Verification items for the finished model (mm, model axes). A direction names the side the tool comes from. Round coordinates to 2 decimals unless told otherwise and drop trailing zeros. Write each loop counter-clockwise with the first axis right and the second up, starting at its lowest first coordinate (ties: lowest second). Pieces come first, ordered by that corner, then holes. Notation, with made-up numbers: M 10,-11 L 56,-11 A20 ccw 56,24 Z; hole C -26,-35.75 d5. An arc over 180 degrees is marked long. Use a Markdown table: item, result. Add a question column.
from build123d import *

# Parameters (mm, degrees)
SKETCH_1_W          = 25
SKETCH_1_H          = 24
EXTRUDE_1_DEPTH     = 1
SKETCH_2_W          = 13
SKETCH_2_H          = 13
EXTRUDE_2_DEPTH     = 3.5
SKETCH_3_R          = 6.5
EXTRUDE_3_DEPTH     = 8.5
SKETCH_4_R          = 5.75
EXTRUDE_4_DEPTH     = 5.5
SKETCH_5_R          = 7
EXTRUDE_5_DEPTH     = 5
SKETCH_6_R          = 0.75
CUT_EXTRUDE_1_DEPTH = 1
SKETCH_7_W          = 14.3
SKETCH_7_H          = 5.5
EXTRUDE_6_DEPTH     = 2


with BuildPart() as part:
    # 草图1 → 凸台-拉伸1 (new body)
    with BuildSketch(Plane.XY):
        Rectangle(SKETCH_1_W, SKETCH_1_H)
    extrude(amount=EXTRUDE_1_DEPTH)

    # 草图2 → 凸台-拉伸2 (add)
    with BuildSketch(Plane.XY.offset(1)):
        with Locations((0, 3.5)):
            Rectangle(SKETCH_2_W, SKETCH_2_H)
    extrude(amount=EXTRUDE_2_DEPTH)

    # 草图3 → 凸台-拉伸3 (add)
    with BuildSketch(Plane.XY.offset(4.5)):
        with Locations((0, 3.5)):
            Circle(SKETCH_3_R)
    extrude(amount=EXTRUDE_3_DEPTH)

    # 草图4 → 凸台-拉伸4 (add)
    with BuildSketch(Plane.XY.offset(13)):
        with Locations((0, 3.5)):
            Circle(SKETCH_4_R)
    extrude(amount=EXTRUDE_4_DEPTH)

    # 草图5 → 凸台-拉伸5 (add)
    with BuildSketch(Plane.XY.offset(18.5)):
        with Locations((0, 3.5)):
            Circle(SKETCH_5_R)
    extrude(amount=EXTRUDE_5_DEPTH)

    # 草图6 → 切除-拉伸1 (cut)
    with BuildSketch(Plane.XY.offset(1)):
        with Locations((10.75, 10.25)):
            Circle(SKETCH_6_R)
        with Locations((10.75, -3.75)):
            Circle(SKETCH_6_R)
        with Locations((-10.75, 10.25)):
            Circle(SKETCH_6_R)
        with Locations((-10.75, -3.75)):
            Circle(SKETCH_6_R)
    extrude(amount=-CUT_EXTRUDE_1_DEPTH, mode=Mode.SUBTRACT)

    # 草图7 → 凸台-拉伸6 (add)
    with BuildSketch(Plane(origin=(0, 0, 0), x_dir=(-1, 0, 0), z_dir=(0, 0, -1))):
        with Locations((0, -9.25)):
            Rectangle(SKETCH_7_W, SKETCH_7_H)
    extrude(amount=EXTRUDE_6_DEPTH)


solid = part.part
1. Cross-section at B-B on y = -9.75. Enter the section's corners in (x, z), plus the area to 3 significant figures.
2. Access from +Z, -Z, +X, -X, +Y, -Y to the whole of each face (thin tool, end or side, straight path). Record for faces 5 (the flat face through (-6.5, 3, 3)), 6 (the flat face through (0, -3, 3)), 7 (the flat face through (-7.15, -9, -1)), 8 (the flat face through (7.15, -9, -1)), 9 (the cylindrical face through (-0.75, 9.2, 15.71)).
3. Cross-section at A-A on x = 10.75. Enter the section's corners in (y, z), plus the area to 3 significant figures.
4. Cross-section at D-D on z = 17. Enter the section's corners in (x, y).
5. Release check for a two-part mould opening along Z. For faces 1 (the flat face through (5, 9, 4.5)), 2 (the flat face through (5, -2, 4.5)), 3 (the flat face through (-12.5, -0.2, 0.5)), 4 (the flat face through (0, -9, -2)) record: +Z half, -Z half, draft (parallel to the pull), parting line (faces both ways), or undercut.
6. Depth check by flat-ended pin: pin 1 Ø3 at (y, z) = (-0.5, 18.5) entering from -X; pin 2 Ø8 at (x, z) = (2, 9) entering from +Y; pin 3 Ø12 at (y, z) = (-6, 11.5) entering from +X. Enter the tip coordinate at first touch or a pass-through.
7. Cross-section at C-C on x = 3.5. Enter the section's corners in (y, z), plus the area to 3 significant figures.
8. Scan lines: line 1 along Y through (x, z) = (-10.75, 0.7); line 2 along Z through (x, y) = (7.25, 2.5); line 3 along Z through (x, y) = (-3.5, 3.25). Record each from-to range of solid material in increasing order. Write a range as from..to.
Answer:
| question | item | result |
|---|---|---|
| 1 | outline | M -12.5,0 L -7.15,0 L -7.15,-2 L 7.15,-2 L 7.15,0 L 12.5,0 L 12.5,1 L -12.5,1 Z |
| 1 | area | 53.6 mm^2 |
| 2 | face 5 | -X, +Y, -Y |
| 2 | face 6 | +X, -X, -Y |
| 2 | face 7 | -Z, -X, +Y, -Y |
| 2 | face 8 | -Z, +X, +Y, -Y |
| 2 | face 9 | none |
| 3 | outline | M -12,0 L -4.5,0 L -4.5,1 L -12,1 Z; M -3,0 L 9.5,0 L 9.5,1 L -3,1 Z; M 11,0 L 12,0 L 12,1 L 11,1 Z |
| 3 | area | 21.0 mm^2 |
| 4 | outline | C 0,3.5 d11.5 |
| 5 | face 1 | undercut |
| 5 | face 2 | undercut |
| 5 | face 3 | draft |
| 5 | face 4 | -Z half |
| 6 | pin 1 | stops at x = -6.54 |
| 6 | pin 2 | stops at y = 10 |
| 6 | pin 3 | stops at x = 5.48 |
| 7 | outline | M -12,-2 L -6.5,-2 L -6.5,0 L 12,0 L 12,1 L 10,1 L 10,4.5 L 8.98,4.5 L 8.98,13 L 8.06,13 L 8.06,18.5 L 9.56,18.5 L 9.56,23.5 L -2.56,23.5 L -2.56,18.5 L -1.06,18.5 L -1.06,13 L -1.98,13 L -1.98,4.5 L -3,4.5 L -3,1 L -12,1 Z |
| 7 | area | 284 mm^2 |
| 8 | line 1 | y = -12..-4.5, -3..9.5, 11..12 |
| 8 | line 2 | z = 0..1 |
| 8 | line 3 | z = 0..23.5 |
